Geometry: final body of the model. Coordinates: model frame, mm. A direction names the side the tool comes from. Coordinates: 2 decimals unless noted, no trailing zeros. Loops run counter-clockwise (first coordinate to the right, second up) from the corner with the lowest first, then second, coordinate; pieces in that order, holes last. Notation, with made-up numbers: (35, 7.25) - (94, 7.25) arc R30 ccw to (94, 42.25) - close; hole circle Ø2 at (79, -24). An arc over 180 degrees is marked (long way). Write each question's results on one line, items separated by ' | '. Start each with the question number.
from build123d import *

# Parameters (mm, degrees)
SKETCH_W        = 74
SKETCH_H        = 102
PAD_DEPTH       = 15
SKETCH001_W     = 72
SKETCH001_H     = 100
SKETCH001_R     = 4.5
SKETCH001_R_2   = 5
SKETCH001_R_3   = 3
POCKET_DEPTH    = 13
SKETCH002_R     = 2
POCKET001_DEPTH = 15.001
POCKET002_DEPTH = 9
SKETCH004_W     = 72
SKETCH004_H     = 100
POCKET003_DEPTH = 3


with BuildPart() as part:
    # Sketch → Pad (new body)
    with BuildSketch(Plane.XY):
        with Locations((37, 51)):
            Rectangle(SKETCH_W, SKETCH_H)
    extrude(amount=PAD_DEPTH)

    # Sketch001 (on Face6 of Pad) → Pocket (cut)
    with BuildSketch(Plane.XY.offset(15)):
        with Locations((37, 51)):
            Rectangle(SKETCH001_W, SKETCH001_H)
        with Locations((67, 25)):
            Circle(SKETCH001_R, mode=Mode.SUBTRACT)
        with Locations((7, 25)):
            Circle(SKETCH001_R, mode=Mode.SUBTRACT)
        with Locations((7, 65)):
            Circle(SKETCH001_R, mode=Mode.SUBTRACT)
        with Locations((67, 65)):
            Circle(SKETCH001_R, mode=Mode.SUBTRACT)
        with Locations((37, 13)):
            Circle(SKETCH001_R_2, mode=Mode.SUBTRACT)
        with Locations((62, 12)):
            Circle(SKETCH001_R_3, mode=Mode.SUBTRACT)
    extrude(amount=-POCKET_DEPTH, mode=Mode.SUBTRACT)

    # Sketch002 (on Face20 of Pocket) → Pocket001 (cut, through all)
    with BuildSketch(Plane.XY.offset(15)):
        with Locations((67, 65)):
            Circle(SKETCH002_R)
        with Locations((67, 25)):
            Circle(SKETCH002_R)
        with Locations((7, 25)):
            Circle(SKETCH002_R)
    extrude(amount=-POCKET001_DEPTH, mode=Mode.SUBTRACT)

    # Sketch003 (on Face4 of Pocket001) → Pocket002 (cut)
    with BuildSketch(Plane(origin=(0, 0, 0), x_dir=(1, 0, 0), z_dir=(0, 0, -1))):
        Polygon((9.75, -26.587713), (9.75, -23.412287), (7, -21.824574), (4.25, -23.412287), (4.25, -26.587713), (7, -28.175426), align=None)
        Polygon((69.75, -26.587713), (69.75, -23.412287), (67, -21.824574), (64.25, -23.412287), (64.25, -26.587713), (67, -28.175426), align=None)
        Polygon((69.75, -66.587713), (69.75, -63.412287), (67, -61.824574), (64.25, -63.412287), (64.25, -66.587713), (67, -68.175426), align=None)
    extrude(amount=-POCKET002_DEPTH, mode=Mode.SUBTRACT)

    # Sketch004 (on Face5 of Pocket002) → Pocket003 (cut)
    with BuildSketch(Plane.XY.offset(15)):
        with Locations((37, 51)):
            Rectangle(SKETCH004_W, SKETCH004_H)
    extrude(amount=-POCKET003_DEPTH, mode=Mode.SUBTRACT)


solid = part.part
1) Pin query (flat end, axial travel): pin 1 Ø3 at (x, y) = (34.5, 66) entering from -Z; pin 2 Ø1.8 at (x, y) = (60.5, 13.5) entering from +Z. Return the tip coordinate at first contact, or that it passes through.
2) Material intervals for line 1 (Y direction, x = 67, z = 10.75); line 2 (Y direction, x = 7, z = 10.7); line 3 (Y direction, x = 67, z = 7.5), sorted ascending. Write a range as [from, to].
3) Section query C-C on x = 56. Output: boundary loops of the cut face in (y, z), and give its area (3 significant figures).
4) Pull-direction query (Y, two-part tool) for faces 4 (the flat face through (65.64, 62.61, 4.44)), 5 (the flat face through (0, 50, 7)); classes: released by +Y, released by -Y, zero draft, split by the parting line, or undercut.
5) Section query D-D on y = 32. Output: boundary loops of the cut face in (x, z), and give its area (3 significant figures).
6) Access query for faces 1 (the flat face through (37, 13, 12)), 2 (the cylindrical face through (5.4, 23.8, 10.5)), 3 (the flat face through (8.36, 27.39, 4.44)). Directions: +Z, -Z, +X, -X, +Y, -Y. A direction counts if a zero-diameter tool reaches every point of the face in a straight line with its end or side. Return the directions, or none.
7) Section query A-A on z = 4.5. Count the separate pieces of the cut face and the enclosed holes in it, and give its area (3 significant figures).
Returned:
1) pin 1: stops at z = 0 | pin 2: stops at z = 12
2) line 1: y = [0, 1], [20.5, 23], [27, 29.5], [60.5, 63], [67, 69.5], [101, 102] | line 2: y = [0, 1], [20.5, 23], [27, 29.5], [60.5, 69.5], [101, 102] | line 3: y = [0, 1], [20.5, 21.82], [28.18, 29.5], [60.5, 61.82], [68.18, 69.5], [101, 102]
3) outline: (0, 0) - (102, 0) - (102, 15) - (101, 15) - (101, 2) - (1, 2) - (1, 15) - (0, 15) - close | area: 230 mm²
4) face 4: undercut | face 5: zero draft
5) outline: (0, 0) - (74, 0) - (74, 15) - (73, 15) - (73, 2) - (1, 2) - (1, 15) - (0, 15) - close | area: 174 mm²
6) face 1: +Z | face 2: +Z, -Z | face 3: -Z
7) separate pieces: 7 | enclosed holes: 4 | area: 631 mm²
